Autodesk Inventor part; units mm, degrees
ref_plane "YZ Plane" through (0, 0, 0) normal (1, 0, 0) x (0, 1, 0)
ref_plane "XZ Plane" through (0, 0, 0) normal (0, 1, 0) x (-1, 0, 0)
ref_plane "XY Plane" through (0, 0, 0) normal (0, 0, 1) x (1, 0, 0)
sketch "Sketch1" plane through (0, 0, 0) normal (0, 0, 1) x (1, 0, 0)
  circle A0 centre (0, 0) radius 46.465
  line L0 (48.75, 10.25) -> (59.25, 10.25)
  line L1 (59.25, 10.25) -> (59.25, -10.25)
  line L2 (59.25, -10.25) -> (48.75, -10.25)
  line L3 (48.75, -10.25) -> (48.75, 10.25)
  circle A1 centre (0, 0) radius 62
  line L4 (59.25, 2) -> (58.75, 2)
  line L5 (58.75, 2) -> (58.75, -2)
  line L6 (58.75, -2) -> (59.25, -2)
  line L7 (59.25, -2) -> (59.25, 2)
  line L8 (54, 10.25) -> (54, -10.25)
  line L9 (48.75, 2) -> (49.25, 2)
  line L10 (49.25, 2) -> (49.25, -2)
  line L11 (49.25, -2) -> (48.75, -2)
  line L12 (48.75, -2) -> (48.75, 2)
  line L13 (27.8929, 52.312) -> (27.6429, 51.879)
  line L14 (31.1071, 49.879) -> (31.3571, 50.312)
  line L15 (31.3571, 50.312) -> (27.8929, 52.312)
  line L16 (27.6429, 51.879) -> (31.1071, 49.879)
  line L17 (22.6429, 43.2187) -> (22.8929, 43.6518)
  line L18 (22.8929, 43.6518) -> (26.3571, 41.6518)
  line L19 (26.1071, 41.2187) -> (22.6429, 43.2187)
  line L20 (26.3571, 41.6518) -> (26.1071, 41.2187)
  line L21 (33.2518, 37.0937) -> (15.4982, 47.3437)
  line L22 (38.5018, 46.187) -> (33.2518, 37.0937)
  line L23 (20.7482, 56.437) -> (38.5018, 46.187)
  line L24 (15.4982, 47.3437) -> (20.7482, 56.437)
  line L25 (-31.3571, 50.312) -> (-31.1071, 49.879)
  line L26 (-27.6429, 51.879) -> (-27.8929, 52.312)
  line L27 (-27.8929, 52.312) -> (-31.3571, 50.312)
  line L28 (-31.1071, 49.879) -> (-27.6429, 51.879)
  line L29 (-26.1071, 41.2187) -> (-26.3571, 41.6518)
  line L30 (-26.3571, 41.6518) -> (-22.8929, 43.6518)
  line L31 (-22.6429, 43.2187) -> (-26.1071, 41.2187)
  line L32 (-22.8929, 43.6518) -> (-22.6429, 43.2187)
  line L33 (-15.4982, 47.3437) -> (-33.2518, 37.0937)
  line L34 (-20.7482, 56.437) -> (-15.4982, 47.3437)
  line L35 (-38.5018, 46.187) -> (-20.7482, 56.437)
  line L36 (-33.2518, 37.0937) -> (-38.5018, 46.187)
  line L37 (-59.25, -2) -> (-58.75, -2)
  line L38 (-58.75, 2) -> (-59.25, 2)
  line L39 (-59.25, 2) -> (-59.25, -2)
  line L40 (-58.75, -2) -> (-58.75, 2)
  line L41 (-48.75, -2) -> (-49.25, -2)
  line L42 (-49.25, -2) -> (-49.25, 2)
  line L43 (-48.75, 2) -> (-48.75, -2)
  line L44 (-49.25, 2) -> (-48.75, 2)
  line L45 (-48.75, 10.25) -> (-48.75, -10.25)
  line L46 (-59.25, 10.25) -> (-48.75, 10.25)
  line L47 (-59.25, -10.25) -> (-59.25, 10.25)
  line L48 (-48.75, -10.25) -> (-59.25, -10.25)
  line L49 (-27.8929, -52.312) -> (-27.6429, -51.879)
  line L50 (-31.1071, -49.879) -> (-31.3571, -50.312)
  line L51 (-31.3571, -50.312) -> (-27.8929, -52.312)
  line L52 (-27.6429, -51.879) -> (-31.1071, -49.879)
  line L53 (-22.6429, -43.2187) -> (-22.8929, -43.6518)
  line L54 (-22.8929, -43.6518) -> (-26.3571, -41.6518)
  line L55 (-26.1071, -41.2187) -> (-22.6429, -43.2187)
  line L56 (-26.3571, -41.6518) -> (-26.1071, -41.2187)
  line L57 (-33.2518, -37.0937) -> (-15.4982, -47.3437)
  line L58 (-38.5018, -46.187) -> (-33.2518, -37.0937)
  line L59 (-20.7482, -56.437) -> (-38.5018, -46.187)
  line L60 (-15.4982, -47.3437) -> (-20.7482, -56.437)
  line L61 (31.3571, -50.312) -> (31.1071, -49.879)
  line L62 (27.6429, -51.879) -> (27.8929, -52.312)
  line L63 (27.8929, -52.312) -> (31.3571, -50.312)
  line L64 (31.1071, -49.879) -> (27.6429, -51.879)
  line L65 (26.1071, -41.2187) -> (26.3571, -41.6518)
  line L66 (26.3571, -41.6518) -> (22.8929, -43.6518)
  line L67 (22.6429, -43.2187) -> (26.1071, -41.2187)
  line L68 (22.8929, -43.6518) -> (22.6429, -43.2187)
  line L69 (15.4982, -47.3437) -> (33.2518, -37.0937)
  line L70 (20.7482, -56.437) -> (15.4982, -47.3437)
  line L71 (38.5018, -46.187) -> (20.7482, -56.437)
  line L72 (33.2518, -37.0937) -> (38.5018, -46.187)
  circle A2 centre (0, 0) radius 49.465
  point P0 (35.8768, 41.6404)
  point P1 (18.1232, 51.8904)
  point P2 (-18.1232, 51.8904)
  point P3 (-35.8768, 41.6404)
  point P4 (-54, 10.25)
  point P5 (-54, -10.25)
  point P6 (-35.8768, -41.6404)
  point P7 (-18.1232, -51.8904)
  point P8 (18.1232, -51.8904)
  point P9 (35.8768, -41.6404)
  dimension "d1" = 92.93
  dimension "d16" = 20.5
  dimension "d17" = 10.5
  dimension "d71" = 54
  dimension "d72" = 10.25
  dimension "d73" = 124
  dimension "d74" = 4
  dimension "d75" = 0.5
  dimension "d76" = 2
  dimension "d83" = 360
  dimension "d85" = 98.93
extrude "Extrusion9" add sketch "Sketch1" along normal blind 7 contours A0 | L0 L8 L2 L3 A2 | L0 L1 L4 L5 L6 L2 L8 | A2 L3 L11 L10 L9 | L3 A2 L69 L67 L57 L55 L45 L43 L33 L31 L21 L19 | L9 L10 L11 L3 | A2 L21 L24 L23 L13 L16 L14 L22 | L21 L20 L18 L17 A2 | L1 L6 L5 L4 | L19 L17 L18 L20 | A2 L69 L68 L66 L65 | L69 L72 L71 L61 L64 L62 L70 A2 | A2 L33 L36 L35 L25 L28 L26 L34 | L33 L32 L30 L29 A2 | L65 L66 L68 L67 | L14 L16 L13 L15 | L31 L29 L30 L32 | A2 L57 L56 L54 L53 | L57 L60 L59 L49 L52 L50 L58 A2 | A2 L45 L48 L47 L37 L40 L38 L46 | L45 L44 L42 L41 A2 | L63 L62 L64 L61 | L53 L54 L56 L55 | L26 L28 L25 L27 | L43 L41 L42 L44 | L51 L50 L52 L49 | L38 L40 L37 L39 | A1
extrude "Extrusion10" add sketch "Sketch1" along normal blind 36 contours A0 | A2 L3 L11 L10 L9 | L3 A2 L69 L67 L57 L55 L45 L43 L33 L31 L21 L19 | L9 L10 L11 L3 | L21 L20 L18 L17 A2 | L19 L17 L18 L20 | A2 L69 L68 L66 L65 | L33 L32 L30 L29 A2 | L65 L66 L68 L67 | L31 L29 L30 L32 | A2 L57 L56 L54 L53 | L45 L44 L42 L41 A2 | L53 L54 L56 L55 | L43 L41 L42 L44
extrude "Extrusion11" cut sketch "Sketch1" along normal blind 36 contours A0
extrude "Extrusion12" cut sketch "Sketch1" along normal blind 7 contours A2 L45 L48 L47 L37 L40 L38 L46 | L45 L44 L42 L41 A2 | L43 L41 L42 L44 | L38 L40 L37 L39
extrude "Extrusion13" add sketch "Sketch1" along normal blind 7 contours L43 L41 L42 L44 | L38 L40 L37 L39
extrude "Extrusion14" add sketch "Sketch1" along normal blind 0.75 contours A2 L45 L48 L47 L37 L40 L38 L46 | L45 L44 L42 L41 A2 | L43 L41 L42 L44 | L38 L40 L37 L39
chamfer "Chamfer4" distance 0.5 angle 45 1 edges at (-58.75, 0, 7)
pattern_circular "Circular Pattern3" count 6 over 360 about axis through (0, 0, 0) along (0, 0, 1) of "Extrusion12", "Extrusion13", "Extrusion14", "Chamfer4"
chamfer "Chamfer5" distance 2.5 angle 45 1 edges at (-46.465, 0, 36)
sketch "Sketch3" plane through (0, 0, 7) normal (0, 0, 1) x (1, 0, 0)
  circle A0 centre (60.75, 0) radius 1
  line L0 (59.25, -2) -> (59.25, 2)
  point P0 (0, 0)
  dimension "d107" = 2
  dimension "d108" = 1.5
extrude "Extrusion15" add sketch "Sketch3" along normal blind 0.5
pattern_circular "Circular Pattern4" count 3 over 360 about axis through (0, 0, 0) along (0, 0, 1) of "Extrusion15"
properties part number "4inchFemale"
Build history of the part. All positions in model axes, mm. A direction names the side the tool comes from. Coordinates: 2 decimals unless noted, no trailing zeros. Order: outer loops, then holes, each group sorted by start corner. A loop starts at its lowest first (then second) coordinate and runs counter-clockwise, first axis right, second up.
Item 1: Tool access for faces 1 (the flat face through (-29.6, 39.2, 3.8)), 2 (the flat face through (-24.371, 54.346, 3.831)): list every direction of +Z, -Z, +X, -X, +Y, -Y with a clear straight run to the whole face (end or side of a thin tool).
Filled in:
face 1: none
face 2: +Z
Item 2: Saw through at B-B on z = 20.5. List the corners of the cut face in (x, y) (3 decimals).
Filled in:
outline: circle Ø98.93 at (0, 0); hole circle Ø92.93 at (0, 0)
Item 3: Saw through at A-A on x = 0. List the corners of the cut face in (y, z) (3 decimals), then the cut area to 3 significant figures.
Filled in:
outline: (-62, 0) - (-46.465, 0) - (-46.465, 33.5) - (-48.965, 36) - (-49.465, 36) - (-49.465, 7) - (-62, 7) - close; (46.465, 0) - (62, 0) - (62, 7) - (49.465, 7) - (49.465, 36) - (48.965, 36) - (46.465, 33.5) - close
area: 385 mm2
Item 4: Saw through at C-C on x = 52. List the corners of the cut face in (y, z), then the cut area to 3 significant figures.
Filled in:
outline: (-33.76, 0) - (33.76, 0) - (33.76, 7) - (10.25, 7) - (10.25, 0.75) - (-10.25, 0.75) - (-10.25, 7) - (-33.76, 7) - close
area: 345 mm2
Item 5: Drop flat-ended pins along their axis: pin 1 Ø5 at (x, z) = (-53.5, 3.5) entering from +Y; pin 2 Ø8 at (x, z) = (23, 11.5) entering from -Y; pin 3 Ø6 at (x, y) = (-38, -24) entering from -Z; pin 4 Ø7 at (y, z) = (-5.5, 4) entering from -X. Give the stop position or say it passes through.
Filled in:
pin 1: stops at y = 35.26
pin 2: stops at y = -45.67
pin 3: stops at z = 0
pin 4: stops at x = -61.97
Item 6: Drill centre lines: L1, parallel to Y at x = 0, z = 24 (3 decimals); L2, parallel to X at y = -1.5, z = 15; L3, parallel to Z at x = -28.5, y = -54. Where is each one in solid material? Low to high.
Filled in:
L1: y = -49.465 to -46.465, 46.465 to 49.465
L2: x = -49.44 to -46.44, 46.44 to 49.44
L3: z = 0 to 7
